For this review, take the finished solid that the model builds, in its own axes (mm). A direction names the side the tool comes from. Give positions to 0.01 mm unless a question says otherwise; leave off trailing zeros. Order: outer loops, then holes, each group sorted by start corner. A loop starts at its lowest first (then second) coordinate and runs counter-clockwise, first axis right, second up.
Item 1: Machinability: for faces 1 (the flat face through (15, 172, 0)), 2 (the flat face through (15, 172, 0.5)), which of the approach directions +Z, -Z, +X, -X, +Y, -Y give a long, thin tool a straight path to every point of the face, cutting with its end or side? Answer none if there is none.
Item 2: Consider section A-A (y = 42.5). Give the boundary of the cut face in (x, z), plus the area to 3 significant figures.
Item 3: Consider section C-C (z = 1.15). Give the boundary of the cut face in (x, y) (3 decimals), plus the area to 3 significant figures.
Item 4: For P1, Ø1.5, axis at x = 8, y = 204.5, coming from the +Z side; P2, Ø0.6, axis at y = 2, z = 0.5, coming from the +X side; P3, Ø2, axis at x = 3.175, y = 335.35, coming from the -Z side, all flat-tipped, find the tip position at first contact; note any pin that passes through.
Item 5: Consider section B-B (x = 18). Give the boundary of the cut face in (y, z) (3 decimals).
Item 6: For probe 1 along X at (y, z) = (335.35, 0.3) (3 decimals); probe 2 along Z at (x, y) = (22.5, 172); probe 3 along X at (y, z) = (335.35, 0.25) (3 decimals), list the stretches that pass through material, from the lowest coordinate up.
Autodesk Inventor part; units mm, degrees
ref_plane "YZ Plane" through (0, 0, 0) normal (1, 0, 0) x (0, 1, 0)
ref_plane "XZ Plane" through (0, 0, 0) normal (0, 1, 0) x (-1, 0, 0)
ref_plane "XY Plane" through (0, 0, 0) normal (0, 0, 1) x (1, 0, 0)
sketch "Sketch1" plane through (0, 0, 0) normal (0, 0, 1) x (1, 0, 0)
  line L0 (0, 0) -> (29.621, 0)
  line L1 (29.621, 0) -> (29.621, 338.525)
  line L2 (29.621, 338.525) -> (0, 338.525)
  line L3 (0, 338.525) -> (0, 0)
  dimension "d0" = 29.621
  dimension "d1" = 338.525
extrude "Plate1" add sketch "Sketch1" along normal blind 0.5
sketch "Sketch2" plane through (30.1974, 338.525, 0.6152) normal (0.3842953, 0, -0.9232102) x (0, 1, 0)
  line L0 (-338.525, 0) -> (0, 0)
  line L1 (0, 0) -> (0, 2.0004)
  line L2 (0, 2.0004) -> (-338.525, 2.0004)
  line L3 (-338.525, 2.0004) -> (-338.525, 0)
edge flange "Flange1" height 2.4 angle 22.6 thickness 0.5 bend radius 1.5 thickness toward (0.3842953, 0, -0.9232102) relief tear relief width 0.5 relief depth 0.25 edges at (29.621, 169.2625, 0.5) wall of the first edge with corners at (30.1974, 0, 0.6152) (30.1974, 338.525, 0.6152) (32.0442, 338.525, 1.3839) (32.0442, 0, 1.3839)
bend "Bend1"
corner "Corner1"
sketch "Sketch3" plane through (0, 0, 0) normal (0, 0, -1) x (-1, 0, 0)
  line L0 (0, 0) -> (-55.5693, 0)
  line L1 (-55.5693, 0) -> (-55.5693, 6.35)
  line L2 (-55.5693, 6.35) -> (0, 6.35)
  line L3 (0, 6.35) -> (0, 0)
  dimension "d13" = 6.35
extrude "Extrusion1" cut sketch "Sketch3" against normal blind 10
sketch "Sketch4" plane through (0, 0, 0) normal (0, 0, -1) x (-1, 0, 0)
  line L0 (0, 6.35) -> (-29.621, 6.35)
  line L1 (-29.621, 6.35) -> (-29.621, 0)
  line L2 (-29.621, 0) -> (0, 0)
  line L3 (0, 0) -> (0, 6.35)
extrude "Extrusion2" add sketch "Sketch4" against normal up to surface (0.5 mm away)
sketch "Sketch5" plane through (0, 0, 0.5) normal (0, 0, 1) x (1, 0, 0)
  line L0 (29.621, 6.35) -> (29.621, 0)
  line L1 (0, 0) -> (0, 3.175) construction
  line L2 (0, 0) -> (0, 338.525) construction
  line L3 (0, 3.175) -> (3.175, 3.175) construction
  line L4 (29.621, 0) -> (29.621, 3.175) construction
  line L5 (29.621, 3.175) -> (26.446, 3.175) construction
  line L6 (3.175, 3.175) -> (3.175, 3.35) construction
  circle A0 centre (3.175, 3.35) radius 1.25
  line L7 (26.446, 3.175) -> (26.446, 3.35) construction
  circle A1 centre (26.446, 3.35) radius 1.25
  dimension "d18" = 3.175
  dimension "d19" = 3.175
  dimension "d20" = 3.175
  dimension "d21" = 3.175
  dimension "d42" = 0.175
  dimension "d43" = 2.5
  dimension "d44" = 0.175
  dimension "d45" = 2.5
extrude "Extrusion3" cut sketch "Sketch5" against normal blind 10
sketch "Sketch6" plane through (0, 0, 0.5) normal (0, 0, 1) x (1, 0, 0)
  line L0 (0, 338.525) -> (0, 335.35) construction
  line L1 (0, 0) -> (0, 338.525) construction
  line L2 (0, 335.35) -> (3.175, 335.35) construction
  line L3 (29.621, 338.525) -> (29.621, 335.35) construction
  line L4 (29.621, 6.35) -> (29.621, 338.525) construction
  line L5 (29.621, 335.35) -> (26.446, 335.35) construction
  circle A0 centre (3.175, 335.35) radius 1.25
  circle A1 centre (26.446, 335.35) radius 1.25
  dimension "d26" = 3.175
  dimension "d27" = 3.175
  dimension "d28" = 3.175
  dimension "d29" = 3.175
  dimension "d34" = 2.5
  dimension "d35" = 2.5
extrude "Extrusion4" cut sketch "Sketch6" against normal blind 10
sketch "Sketch7" plane through (0, 0, 0.5) normal (0, 0, 1) x (1, 0, 0)
  line L0 (29.621, 6.35) -> (29.621, 0)
  line L1 (29.621, 6.35) -> (33.3489, 6.35)
  line L2 (33.3489, 6.35) -> (33.3489, 6.525)
  line L3 (33.3489, 6.525) -> (29.621, 6.525)
  line L4 (29.621, 6.525) -> (29.621, 6.35)
  line L5 (29.621, 0) -> (-2.8876, 0)
  line L6 (-2.8876, 0) -> (-2.8876, 0.175)
  line L7 (-2.8876, 0.175) -> (29.621, 0.175)
  line L8 (29.621, 0.175) -> (29.621, 0)
  dimension "d36" = 0.175
  dimension "d37" = 0.175
extrude "Extrusion5" cut sketch "Sketch7" against normal blind 10 and the other way blind 5
equation "\"d2\" = Thickness"
equation "\"d3\" = BendReliefWidth"
equation "\"d4\" = BendReliefDepth"
equation "\"d5\" = MinimumRemnant"
equation "\"d6\" = TransitionRadius"
equation "\"d10\" = CornerReliefSize"
equation "\"d11\" = GapSize"
equation "\"d12\" = JacobiRadiusSize"
equation "\"BendRadius\" = Thickness"
equation "\"BendReliefWidth\" = Thickness"
equation "\"BendReliefDepth\" = 0.5 * Thickness"
equation "\"CornerReliefSize\" = 4 * Thickness"
equation "\"MinimumRemnant\" = 2 * Thickness"
equation "\"TransitionRadius\" = BendRadius"
equation "\"JacobiRadiusSize\" = BendRadius"
equation "\"GapSize\" = Thickness"
properties part number "sideplate part 2 mirror"
Resolved:
1. face 1: -Z, +X, -X, +Y, -Y
1. face 2: +Z, -X, +Y, -Y
2. outline: (0, 0) - (29.62, 0) arc R2 ccw to (30.39, 0.15) - (32.24, 0.92) - (32.04, 1.38) - (30.2, 0.62) arc R1.5 cw to (29.62, 0.5) - (0, 0.5) - close
2. area: 16.2 mm2
3. outline: (31.482, 6.525) - (32.142, 6.525) - (32.142, 338.525) - (31.482, 338.525) - close
3. area: 219 mm2
4. P1: stops at z = 0.5
4. P2: stops at x = 29.62
4. P3: passes through
5. outline: (0.175, 0) - (338.525, 0) - (338.525, 0.5) - (0.175, 0.5) - close
6. probe 1: x = 0 to 1.925, 4.425 to 25.196, 27.696 to 30.741
6. probe 2: z = 0 to 0.5
6. probe 3: x = 0 to 1.925, 4.425 to 25.196, 27.696 to 30.621
